Here's how the part is built. I have some questions about the finished solid (model axes, mm). A direction names the side the tool comes from. Coordinates: 2 decimals unless noted, no trailing zeros. Loops run counter-clockwise (first coordinate to the right, second up) from the corner with the lowest first, then second, coordinate; pieces in that order, holes last. Notation, with made-up numbers: M 84.25,17.25 L 122.25,17.25 A9 cw 122.25,30.25 Z; hole C 59,-7 d4. An arc over 180 degrees is marked long. Use CSV: the item, a comma, the result in double quotes. Start each with the question number.
Q1. Please list where these lines run through material, in increasing order: probe 1 along X at (y, z) = (-8, 4); probe 2 along Y at (x, z) = (-1.5, 2.75); probe 3 along X at (y, z) = (-6.25, 1.5). Write a range as [from, to].
Q2. If we section it at C-C (x = -4.5): Please give me the cut outline in (y, z), and give its area (3 significant figures).
Q3. If we section it at B-B (z = 5.25): Please give me the cut outline in (x, y).
Q4. If we section it at A-A (y = -6.5): Please give me the cut outline in (x, z), and give its area (3 significant figures).
Q5. If we section it at D-D (z = 1): Please give me the cut outline in (x, y).
Q6. Which directions (+Z, -Z, +X, -X, +Y, -Y) give clear straight access to the entire face, cutting with the end or side of a thin tool? Please do faces 1 (the flat face through (-8.42, -4, 4)), 2 (the flat face through (0, -2.25, 4)).
Q7. If we mould it in two halves opening along X, with no side actions, what happens to faces 3 (the flat face through (8.42, -4, 4)), 4 (the cylindrical face through (4.5, -6.3, 0.7)), 5 (the flat face through (-2, -10.25, 8))? For each: +X half, -X half, draft (parallel to the pull), parting line (faces both ways), or undercut.
from build123d import *

# Parameters (mm, degrees)
SKETCH1_W           = 16.84
SKETCH1_H           = 12
BOSS_EXTRUDE1_DEPTH = 8.4
CUT_EXTRUDE1_DEPTH  = 8


with BuildPart() as part:
    # Sketch1 → Boss-Extrude1 (new body)
    with BuildSketch(Plane.XY):
        with Locations((0, -4.25)):
            Rectangle(SKETCH1_W, SKETCH1_H)
    extrude(amount=BOSS_EXTRUDE1_DEPTH)

    # Sketch2 → Cut-Extrude1 (cut)
    with BuildSketch(Plane.XZ.offset(10.25)):
        with BuildLine():
            Line((7.42, 6.9), (-7.42, 6.9))
            Line((-7.42, 6.9), (-7.42, 1.7))
            Line((-7.42, 1.7), (-6.82, 1.7))
            ThreePointArc((-6.82, 1.7), (-4.546666667, 0.7), (-2.273333333, 1.7))
            ThreePointArc((-2.273333333, 1.7), (0, 0.7), (2.273333333, 1.7))
            ThreePointArc((2.273333333, 1.7), (4.546666667, 0.7), (6.82, 1.7))
            Line((6.82, 1.7), (7.42, 1.7))
            Line((7.42, 1.7), (7.42, 6.9))
        make_face()
    extrude(amount=-CUT_EXTRUDE1_DEPTH, mode=Mode.SUBTRACT)


solid = part.part
Results below:
1,probe 1,"[-8.42, -7.42], [7.42, 8.42]"
1,probe 2,"[-2.25, 1.75]"
1,probe 3,"[-8.42, -6.62], [-2.47, -2.07], [2.07, 2.47], [6.62, 8.42]"
2,outline,"M -10.25,0 L 1.75,0 L 1.75,8.4 L -10.25,8.4 L -10.25,6.9 L -2.25,6.9 L -2.25,0.7 L -10.25,0.7 Z"
2,area,"51.2 mm^2"
3,outline,"M -8.42,-10.25 L -7.42,-10.25 L -7.42,-2.25 L 7.42,-2.25 L 7.42,-10.25 L 8.42,-10.25 L 8.42,1.75 L -8.42,1.75 Z"
4,outline,"M -8.42,0 L 8.42,0 L 8.42,8.4 L -8.42,8.4 Z; hole M -7.42,1.7 L -6.82,1.7 A3.08 ccw -2.27,1.7 A3.08 ccw 2.27,1.7 A3.08 ccw 6.82,1.7 L 7.42,1.7 L 7.42,6.9 L -7.42,6.9 Z"
4,area,"54.9 mm^2"
5,outline,"M -8.42,-10.25 L -5.87,-10.25 L -5.87,-2.25 L -3.22,-2.25 L -3.22,-10.25 L -1.33,-10.25 L -1.33,-2.25 L 1.33,-2.25 L 1.33,-10.25 L 3.22,-10.25 L 3.22,-2.25 L 5.87,-2.25 L 5.87,-10.25 L 8.42,-10.25 L 8.42,1.75 L -8.42,1.75 Z"
6,face 1,"+Z, -Z, -X, +Y, -Y"
6,face 2,"-Y"
7,face 3,"+X half"
7,face 4,"undercut"
7,face 5,"draft"
